Design review of the part built by this model. Coordinates are the model's own, in mm. Round coordinates to 2 decimals unless told otherwise and drop trailing zeros. Order: outer loops, then holes, each group sorted by start corner. A loop starts at its lowest first (then second) coordinate and runs counter-clockwise, first axis right, second up. Notation, with made-up numbers: (34, 79.5) - (44, 79.5) arc R33 cw to (44, 114.5) - close; hole circle Ø2 at (-2, 80.5). An arc over 180 degrees is marked (long way). Write item = value, one per line.
from build123d import *

# Parameters (mm, degrees)
BOSS_EXTRUDE1_DEPTH = 228.6
SKETCH3_R           = 2.413
CUT_EXTRUDE1_DEPTH  = 1.905
LPATTERN1_COUNT     = 3
LPATTERN1_PITCH     = 76.2


with BuildPart() as part:
    # Sketch2 → Boss-Extrude1 (new, symmetric)
    with BuildSketch(Plane(origin=(0, 0, 0), x_dir=(0, 0, -1), z_dir=(1, 0, 0))):
        Polygon((0, 9.144), (-12.192, 9.144), (-12.192, 4.445), (-10.6045, 4.445), (-10.6045, 5.969), (-4.2545, 5.969), (-4.2545, 4.445), (-1.905, 4.445), (-1.905, -4.445), (-4.2545, -4.445), (-4.2545, -5.969), (-10.6045, -5.969), (-10.6045, -4.445), (-12.192, -4.445), (-12.192, -9.144), (0, -9.144), align=None)
    extrude(amount=BOSS_EXTRUDE1_DEPTH, both=True)

    # Sketch3 → Cut-Extrude1 (cut)
    with BuildSketch(Plane.XY.offset(1.905)):
        with Locations((38.1, 0)):
            Circle(SKETCH3_R)
    cut_extrude1 = extrude(amount=-CUT_EXTRUDE1_DEPTH, mode=Mode.SUBTRACT)

    # LPattern1: Cut-Extrude1 ×3
    with Locations(*[(i * LPATTERN1_PITCH, 0, 0) for i in range(1, LPATTERN1_COUNT)]):
        add(cut_extrude1, mode=Mode.SUBTRACT)

    # SurfaceCut1
    split(bisect_by=Plane(origin=(0, 0, 0), x_dir=(0, 0, -1), z_dir=(1, 0, 0)), keep=Keep.TOP)

    # Mirror1: part across plane


with BuildPart() as part_1:
    add(part.part)
    add(part.part.mirror(Plane(origin=(0, 0, 0), x_dir=(0, 0, 1), z_dir=(1, 0, 0))))


solid = part_1.part
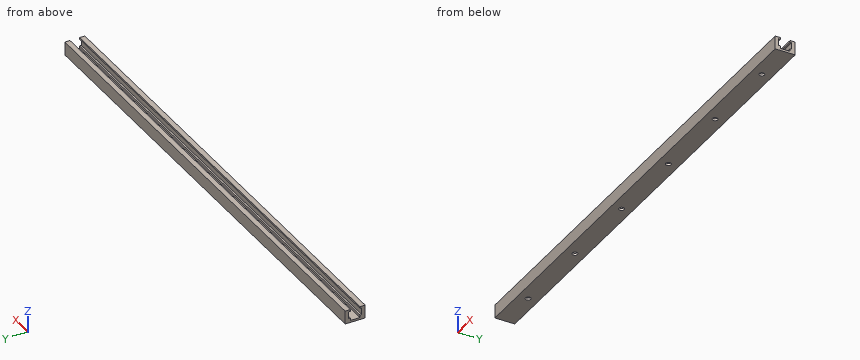
1) Clearance check with flat-ended pins moving along their axes: pin 1 Ø10 at (x, y) = (-86, 6.5) entering from -Z; pin 2 Ø4.5 at (x, y) = (100.5, 1) entering from +Z (3 decimals); pin 3 Ø4 at (x, y) = (-38.1, 0) entering from +Z (3 decimals). State where each tip first meets the part, or that it passes through.
Findings:
pin_1 = 0
pin_2 = 1.905
pin_3 = through
2) We need section A-A on z = 7.5. Write out the cut boundary in (x, y), and give its area (3 significant figures).
Findings:
outline = (-228.6, -9.14) - (228.6, -9.14) - (228.6, -5.97) - (-228.6, -5.97) - close; (-228.6, 5.97) - (228.6, 5.97) - (228.6, 9.14) - (-228.6, 9.14) - close
area = 2,900 mm^2
3) To check wall thickness, follow L1, parallel to Y at x = -16, z = 10.25; L2, parallel to Y at x = 114.3, z = 0.6; L3, parallel to Z at x = 134.5, y = 2.5 (3 decimals). State the ranges of each line that lie inside material, in increasing order. Write a range as from..to.
Findings:
L1 = -9.14..-5.97, 5.97..9.14
L2 = -9.14..-2.41, 2.41..9.14
L3 = 0..1.905
4) We need section B-B on x = -144.5. Write out the cut boundary in (y, z) (1 decimal), and give its area (3 significant figures).
Findings:
outline = (-9.1, 0) - (9.1, 0) - (9.1, 12.2) - (4.4, 12.2) - (4.4, 10.6) - (6, 10.6) - (6, 4.3) - (4.4, 4.3) - (4.4, 1.9) - (-4.4, 1.9) - (-4.4, 4.3) - (-6, 4.3) - (-6, 10.6) - (-4.4, 10.6) - (-4.4, 12.2) - (-9.1, 12.2) - close
area = 112 mm^2
